```python
from build123d import *

# Parameters (mm, degrees)
FILLET2_R              = 10.795
F_1_1_DIAMETER_HOLE1_D = 25.4


with BuildPart() as part:
    # Sketch1 → Revolve1 (revolve)
    with BuildSketch(Plane.XY, mode=Mode.PRIVATE) as revolve1_sk:
        Polygon((87.63, 0), (57.15, 0), (57.15, 7.0866), (0, 7.0866), (0, 17.2466), (57.15, 17.2466), (57.15, 31.75), (87.63, 31.75), align=None)
    revolve(revolve1_sk.sketch.rotate(Axis((0, 7.0866, 0), (0, 1, 0)), 90), axis=Axis((0, 7.0866, 0), (0, 1, 0)))

    # Fillet2
    # the kernel refuses this fillet: 10.795 mm, written as the material it adds along each edge
    with BuildSketch(Plane(origin=(0, 17.2466, 0), x_dir=(0, 0, -1), z_dir=(1, 0, 0))) as fillet2_piece_1:
        with BuildLine():
            CenterArc((57.15 - FILLET2_R, FILLET2_R), FILLET2_R, 270, 90)
            Line((57.15, FILLET2_R), (57.15 + FILLET2_R * 0.02, FILLET2_R))
            Line((57.15 + FILLET2_R * 0.02, FILLET2_R), (57.15 + FILLET2_R * 0.02, -FILLET2_R * 0.02))
            Line((57.15 + FILLET2_R * 0.02, -FILLET2_R * 0.02), (57.15 - FILLET2_R, -FILLET2_R * 0.02))
            Line((57.15 - FILLET2_R, -FILLET2_R * 0.02), (57.15 - FILLET2_R, 0))
        make_face()
    revolve(axis=Axis((0, 17.2466, 0), (0, 1, 0)))
    with BuildSketch(Plane(origin=(0, 7.0866, 0), x_dir=(0, 0, -1), z_dir=(1, 0, 0))) as fillet2_piece_2:
        with BuildLine():
            CenterArc((47.011962989, -10.795), FILLET2_R, 20.092051419, 69.907948581)
            Line((47.011962989, 0), (47.011962989, 0.2159))
            Line((47.011962989, 0.2159), (57.15, 0.2159))
            Line((57.15, 0.2159), (57.3659, 0))
            ThreePointArc((57.3659, 0), (57.3659, -3.5433), (57.35276074, -7.012432))
            Line((57.35276074, -7.012432), (57.15, -7.0866))
        make_face()
    revolve(axis=Axis((0, 7.0866, 0), (0, 1, 0)))

    # 1 (1) Diameter Hole1 (through all)
    with Locations(Plane(origin=(0, 17.2466, 0), x_dir=(1, 0, 0), z_dir=(0, 1, 0))):
        with Locations((0, 0)):
            Hole(F_1_1_DIAMETER_HOLE1_D / 2)


solid = part.part
```
Source: CAD feature listing. Evaluate the final solid. Frame: model axes, mm. A direction names the side the tool comes from. Give positions to 0.01 mm unless a question says otherwise; leave off trailing zeros. Order: outer loops, then holes, each group sorted by start corner. A loop starts at its lowest first (then second) coordinate and runs counter-clockwise, first axis right, second up.
(1) Pull-direction query (X, two-part tool) for faces 3 (the face through (57, 31.75, 18)), 4 (the face through (85.546, 15.653, 18.996)), 5 (the face through (10, 17.247, 10)), 6 (the face through (-2.513, 29.922, 57.095)); classes: +X half, -X half, draft (parallel to the pull), parting line (faces both ways), or undercut.
(2) Material intervals for line 1 along X through (y, z) = (30.45, 0); line 2 along X through (y, z) = (21.5, 32); line 3 along Y through (x, z) = (4, -46.5), sorted ascending.
(3) Section query A-A (x = 0). Return the cut outline in (y, z) (3 decimals).
(4) Section query D-D (z = 64). Return the cut outline in (x, y).
(5) Section query C-C (y = 14.5). Return the cut outline in (x, z), plus the area to 3 significant figures.
(6) Access query for faces 1 (the face through (2.75, 12.1, 12.4)), 2 (the face through (10, 7.087, -10)). Directions: +Z, -Z, +X, -X, +Y, -Y. A direction counts if a zero-diameter tool reaches every point of the face in a straight line with its end or side. Return the directions, or none.
(7) Section query B-B (z = 0). Return the cut outline in (x, y) (3 decimals), plus the area to 3 significant figures.
(8) Contact query for flat-ended pins moving along their axis: P1, Ø12, axis at x = 53, y = 21, coming from the +Z side; P2, Ø10, axis at x = 7, z = 45, coming from the +Y side; P3, Ø8, axis at x = 55, y = 19.5, coming from the -Z side. Output: stop coordinate, or through.
Outcome:
1. face 3: draft
1. face 4: parting line
1. face 5: undercut
1. face 6: undercut
2. line 1: x = -87.63 to -57.15, 57.15 to 87.63
2. line 2: x = -81.58 to -44.66, 44.66 to 81.58
2. line 3: y = 7.09 to 17.25
3. outline: (0, -87.63) - (31.75, -87.63) - (31.75, -57.15) - (28.042, -57.15) arc R10.795 cw to (17.247, -46.355) - (17.247, -12.7) - (7.087, -12.7) - (7.087, -47.012) arc R10.795 cw to (0, -57.15) - close; (0, 57.15) arc R10.795 cw to (7.087, 47.012) - (7.087, 12.7) - (17.247, 12.7) - (17.247, 46.355) arc R10.795 cw to (28.042, 57.15) - (31.75, 57.15) - (31.75, 87.63) - (0, 87.63) - close
4. outline: (-59.86, 0) - (59.86, 0) - (59.86, 31.75) - (-59.86, 31.75) - close
5. outline: circle Ø175.26 at (0, 0); hole circle Ø25.4 at (0, 0)
5. area: 23,600 mm2
6. face 1: +Y, -Y
6. face 2: -Y
7. outline: (-87.63, 0) - (-57.15, 0) arc R10.795 cw to (-47.012, 7.087) - (-12.7, 7.087) - (-12.7, 17.247) - (-46.355, 17.247) arc R10.795 cw to (-57.15, 28.042) - (-57.15, 31.75) - (-87.63, 31.75) - close; (12.7, 7.087) - (47.012, 7.087) arc R10.795 cw to (57.15, 0) - (87.63, 0) - (87.63, 31.75) - (57.15, 31.75) - (57.15, 28.042) arc R10.795 cw to (46.355, 17.247) - (12.7, 17.247) - close
7. area: 2,930 mm2
8. P1: stops at z = 73.96
8. P2: stops at y = 18.09
8. P3: stops at z = -71.26
